Solid Edge part; units mm, degrees
sketch "Sketch1" plane through (0, 0, 0) normal (1, 0, 0) x (0, 1, 0)
  line L0 (0, 30) -> (80, 30)
  line L1 (80, 30) -> (80, 25)
  line L2 (80, 25) -> (83, 25)
  line L3 (83, 25) -> (83, 5)
  line L4 (83, 5) -> (80, 5)
  line L5 (80, 5) -> (80, 0)
  line L6 (80, 0) -> (0, 0)
  line L7 (0, 0) -> (0, 5)
  line L8 (0, 5) -> (-3, 5)
  line L9 (-3, 5) -> (-3, 25)
  line L10 (-3, 25) -> (0, 25)
  line L11 (0, 25) -> (0, 30)
  dimension "D1" = 3
  dimension "D2" = 3
extrude "Protrusion1" add sketch "Sketch1" against normal blind 3
properties material "Acier"
Design review of the part built by this model. Coordinates are the model's own, in mm. A direction names the side the tool comes from. Give positions to 0.01 mm unless a question says otherwise; leave off trailing zeros. Order: outer loops, then holes, each group sorted by start corner. A loop starts at its lowest first (then second) coordinate and runs counter-clockwise, first axis right, second up. Notation, with made-up numbers: (-2, -29) - (17, -29) arc R25 ccw to (17, 2) - close; hole circle Ø8 at (18, 22). An arc over 180 degrees is marked (long way). Write item = value, one per line. Start each with the question number.
Q1. To check wall thickness, follow L1, parallel to Y at x = -2.4, z = 26.75. State the ranges of the line that lie inside material, in increasing order. Write a range as from..to.
Q2. We need section A-A on x = -1.9. State the section outline as (y, z) points, plus the area to 3 significant figures.
Q3. Tool access review of faces 1 (the face through (-1, 80, 28)), 2 (the face through (0, 39, 15)), 3 (the face through (-1, -1, 5)), 4 (the face through (-1, 82, 5)), 5 (the face through (-1, -2, 25)): name each direction out of +Z, -Z, +X, -X, +Y, -Y from which nothing blocks a thin tool from reaching the whole face with its end or side.
Q4. Clearance check with flat-ended pins moving along their axes: pin 1 Ø0.9 at (x, y) = (-2, -2) entering from -Z; pin 2 Ø1.5 at (x, y) = (-2, 81.5) entering from +Z; pin 3 Ø1.5 at (x, z) = (-1, 26.5) entering from -Y. State where each tip first meets the part, or that it passes through.
Working result:
q1.L1 = 0..80
q2.outline = (-3, 5) - (0, 5) - (0, 0) - (80, 0) - (80, 5) - (83, 5) - (83, 25) - (80, 25) - (80, 30) - (0, 30) - (0, 25) - (-3, 25) - close
q2.area = 2,520 mm²
q3.face_1 = +Z, +X, -X, +Y
q3.face_2 = +Z, -Z, +X, +Y, -Y
q3.face_3 = -Z, +X, -X, -Y
q3.face_4 = -Z, +X, -X, +Y
q3.face_5 = +Z, +X, -X, -Y
q4.pin_1 = 5
q4.pin_2 = 25
q4.pin_3 = 0
